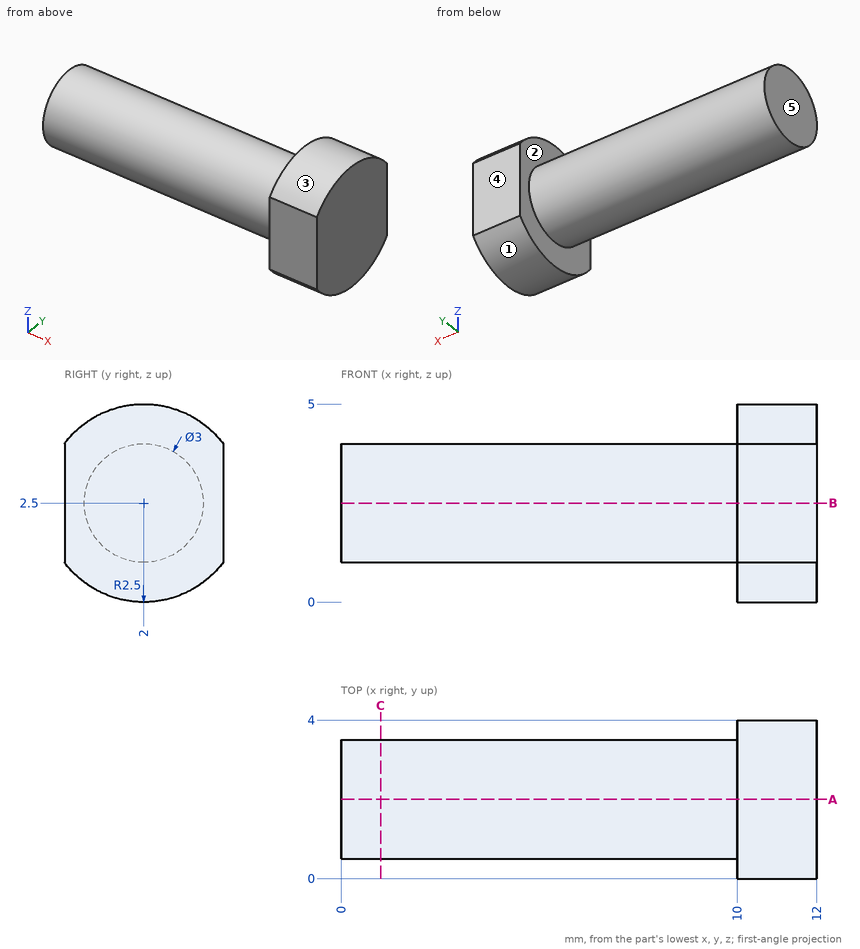
For this review, use the dimensioned drawing (mm, ordinates from the lowest corner) and the shaded views. A direction names the side the tool comes from. Round coordinates to 2 decimals unless told otherwise and drop trailing zeros. Loops run counter-clockwise (first coordinate to the right, second up) from the corner with the lowest first, then second, coordinate; pieces in that order, holes last. Notation, with made-up numbers: M 34,-14 L 86,-14 A32 cw 86,25 Z; hole C 56,37 d9. An arc over 180 degrees is marked long. Answer as a JSON object with one key per item and string values.
(1) Take a section at C-C on x = 1. Give the boundary of the cut face in (y, z), and give its area (3 significant figures).
Resolved:
{"outline": "C 2,2.5 d3", "area": "7.07 mm²"}
(2) Clearance check with a flat-ended pin moving along its axis: P1, Ø1, axis at x = 8, y = 2, coming from the +Z side. State where the tip first meets the part, or that it passes through.
Resolved:
{"P1": "z = 4"}
(3) To check wall thickness, follow line 1 along X through (y, z) = (0.45, 4.2); line 2 along Z through (x, y) = (7, 2.05); line 3 along Z through (x, y) = (11.75, 3.15). State the ranges of each line that lie inside material, in increasing order.
Resolved:
{"line 1": "10 to 12", "line 2": "1 to 4", "line 3": "0.28 to 4.72"}
(4) Take a section at A-A on y = 2. Give the boundary of the cut face in (x, z), and give its area (3 significant figures).
Resolved:
{"outline": "M 0,1 L 10,1 L 10,0 L 12,0 L 12,5 L 10,5 L 10,4 L 0,4 Z", "area": "40.0 mm²"}
(5) Draft analysis for pull direction Y (two halves, no side actions). For the marked faces 3, 4 and 5, state which applies: released by +Y, released by -Y, zero draft, split by the parting line, or undercut.
Resolved:
{"face 3": "split by the parting line", "face 4": "released by +Y", "face 5": "zero draft"}
(6) Take a section at B-B on z = 2.5. Give the boundary of the cut face in (x, y).
Resolved:
{"outline": "M 0,0.5 L 10,0.5 L 10,0 L 12,0 L 12,4 L 10,4 L 10,3.5 L 0,3.5 Z"}
(7) Tool access review of the marked faces 1 and 2: name each direction out of +Z, -Z, +X, -X, +Y, -Y from which nothing blocks a thin tool from reaching the whole face with its end or side.
Resolved:
{"face 1": "-Z, +X, -X", "face 2": "-X"}
